For this review, use the dimensioned drawing (mm, ordinates from the lowest corner) and the shaded views. A direction names the side the tool comes from. Give positions to 0.01 mm unless a question says otherwise; leave off trailing zeros. Order: outer loops, then holes, each group sorted by start corner. A loop starts at its lowest first (then second) coordinate and runs counter-clockwise, first axis right, second up. Notation, with made-up numbers: (33.5, -29.75) -> (72.5, -29.75) arc R19 ccw to (72.5, -22.75) -> close; hole circle Ø10 at (4, 53). An arc over 180 degrees is marked (long way). Return JSON: item names as keys, results as strings.
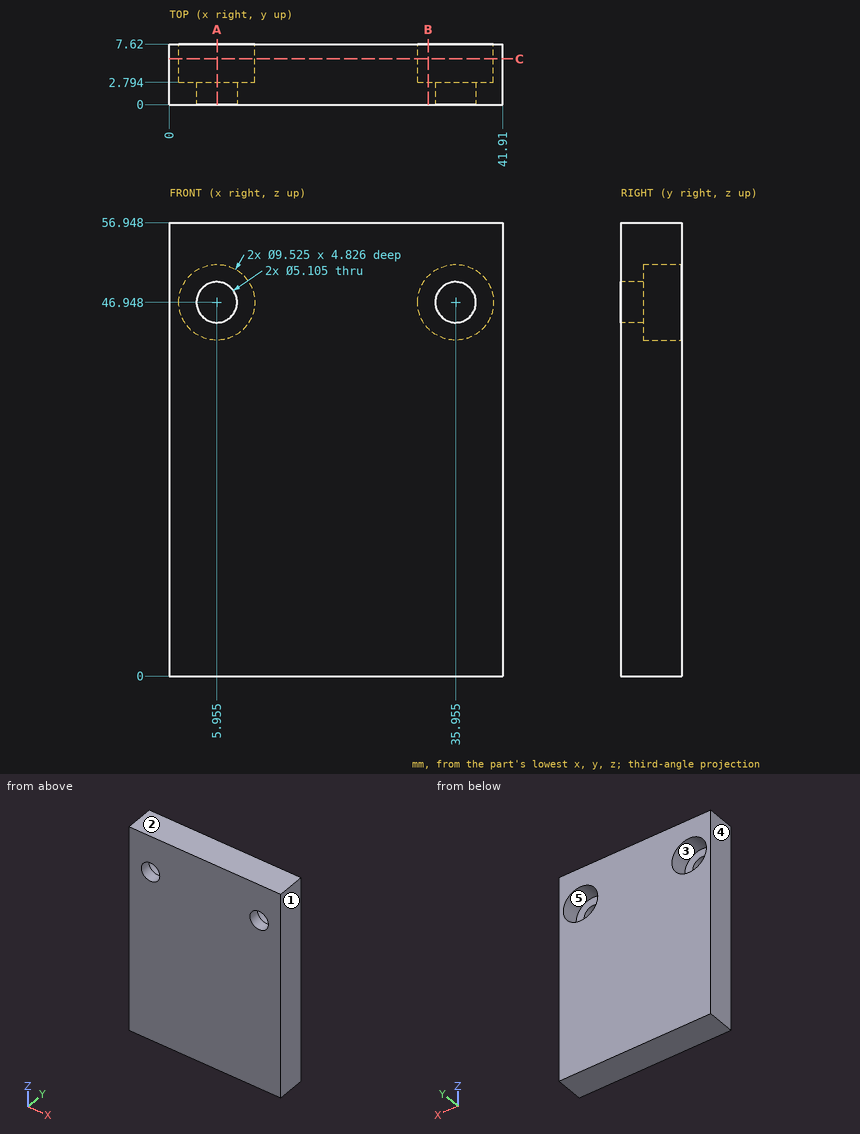
Item 1: For pin 1 (6.5 mm diameter, centred on x = 5.96, z = 46.95, fed in from +Y), flat-tipped, find the tip position at first contact; note if it passes through.
Result set:
{"pin 1": "stops at y = 2.79"}
Item 2: Add section B-B (x = 32.5). Give the boundary of the cut face in (y, z) (1 decimal).
Result set:
{"outline": "(0, 0) -> (7.6, 0) -> (7.6, 43.7) -> (2.8, 43.7) -> (2.8, 50.2) -> (7.6, 50.2) -> (7.6, 56.9) -> (0, 56.9) -> close"}
Item 3: Add section A-A (x = 6). Give the boundary of the cut face in (y, z) (1 decimal), plus the area to 3 significant figures.
Result set:
{"outline": "(0, 0) -> (7.6, 0) -> (7.6, 42.2) -> (2.8, 42.2) -> (2.8, 44.4) -> (0, 44.4) -> close; (0, 49.5) -> (2.8, 49.5) -> (2.8, 51.7) -> (7.6, 51.7) -> (7.6, 56.9) -> (0, 56.9) -> close", "area": "374 mm^2"}
Item 4: Mouldability with a two-part tool opening along X and no side actions: class the marked faces 1, 2 and 3 as released by +X, released by -X, zero draft, split by the parting line, or undercut.
Result set:
{"face 1": "released by +X", "face 2": "zero draft", "face 3": "undercut"}
Item 5: Wall thickness on L1, parallel to X at y = 4, z = 45.5; L2, parallel to X at y = 7, z = 44.5; L3, parallel to Z at x = 33.5, y = 6.5 (1 decimal): over which ranges is each line inside the solid? List them lowest first. Write a range as [from, to].
Result set:
{"L1": "x = [0, 1.42], [10.49, 31.42], [40.49, 41.91]", "L2": "x = [0, 1.87], [10.04, 31.87], [40.04, 41.91]", "L3": "z = [0, 42.9], [51, 56.9]"}
Item 6: Machinability: for the marked faces 4 and 5, which of the approach directions +Z, -Z, +X, -X, +Y, -Y give a long, thin tool a straight path to every point of the face, cutting with its end or side? Answer none if there is none.
Result set:
{"face 4": "+Z, -Z, -X, +Y, -Y", "face 5": "+Y"}
Item 7: Add section C-C (y = 5.75). Give the boundary of the cut face in (x, z) (1 decimal).
Result set:
{"outline": "(0, 0) -> (41.9, 0) -> (41.9, 56.9) -> (0, 56.9) -> close; hole circle Ø9.5 at (6, 46.9); hole circle Ø9.5 at (36, 46.9)"}
